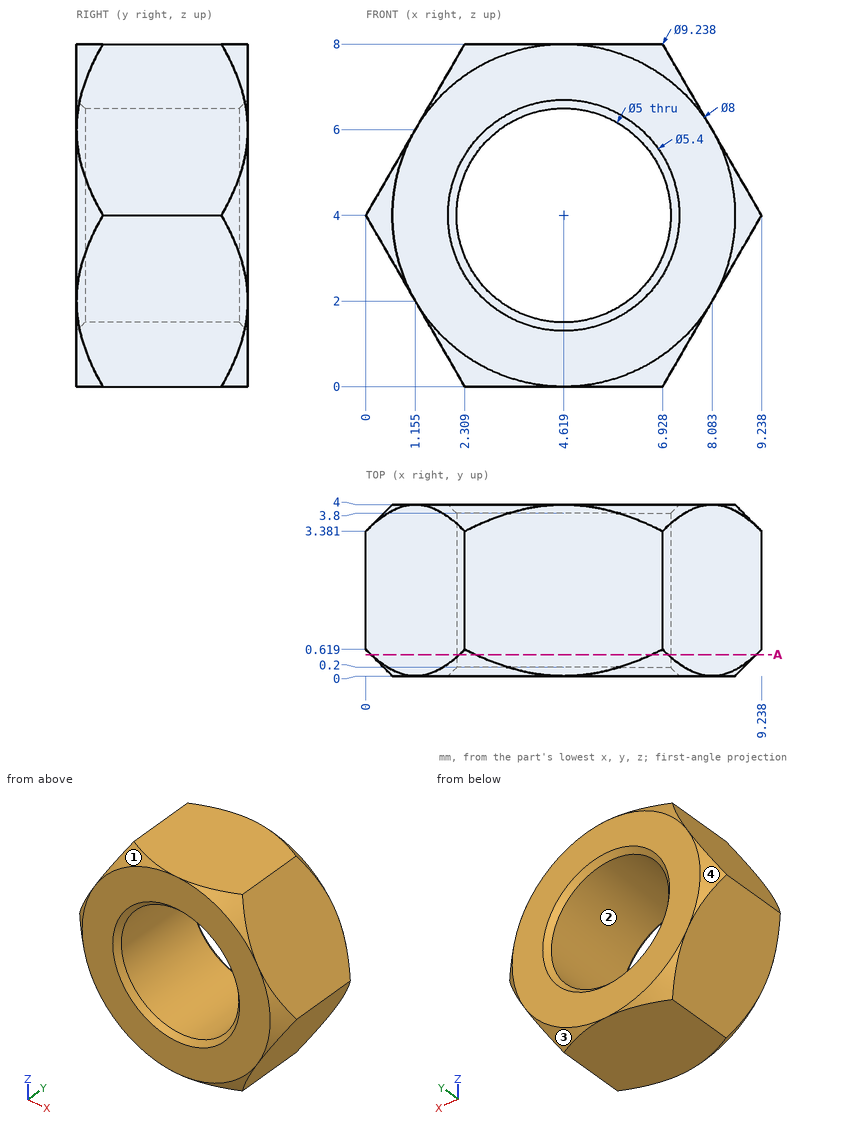
Verification items for this drawing (mm, ordinates from the low corner). Round coordinates to 2 decimals unless told otherwise and drop trailing zeros. Write each loop counter-clockwise with the first axis right and the second up, starting at its lowest first coordinate (ties: lowest second). Pieces come first, ordered by that corner, then holes. Notation, with made-up numbers: (14, 44) - (22, 44) arc R26 cw to (22, 75) - close; hole circle Ø11 at (-14, 76.25). An arc over 180 degrees is marked (long way). Answer as a JSON object with one key per item and string values. Group by question number.
Q1. Section check A-A, the plane y = 0.5. Enter the section's corners in (x, z) (1 decimal).
Q2. Mould release check, pull along Z, two halves, no side actions. Record for the marked faces 1, 2, 3 and 4: released by +Z, released by -Z, zero draft, split by the parting line, or undercut.
Q3. Go/stop test with flat-tipped pins: pin 1 Ø1.5 at (y, z) = (1, 2) entering from +X (1 decimal); pin 2 Ø3 at (x, z) = (4.62, 4) entering from +Y. Record where each tip stops, or that it passes through.
Q4. Thickness scan on line 1 (Z direction, x = 3.5, y = 1.1) (1 decimal); line 2 (Z direction, x = 4.25, y = 1.8); line 3 (X direction, y = 1.5, z = 4.75) (1 decimal). Record the ranges inside material, lowest first.
Found:
{
 "1": {"outline": "(0.1, 3.8) - (2.2, 0.2) arc R4.5 ccw to (2.6, 0) - (6.7, 0) arc R4.5 ccw to (7.1, 0.2) - (9.1, 3.8) arc R4.5 ccw to (9.1, 4.2) - (7.1, 7.8) arc R4.5 ccw to (6.7, 8) - (2.6, 8) arc R4.5 ccw to (2.2, 7.8) - (0.1, 4.2) arc R4.5 ccw to start; hole circle Ø5 at (4.6, 4)"},
 "2": {"face 1": "released by +Z", "face 2": "undercut", "face 3": "released by -Z", "face 4": "split by the parting line"},
 "3": {"pin 1": "stops at x = 8.5", "pin 2": "passes through"},
 "4": {"line 1": "z = 0 to 1.8, 6.2 to 8", "line 2": "z = 0 to 1.53, 6.47 to 8", "line 3": "x = 0.4 to 2.2, 7 to 8.8"}
}
